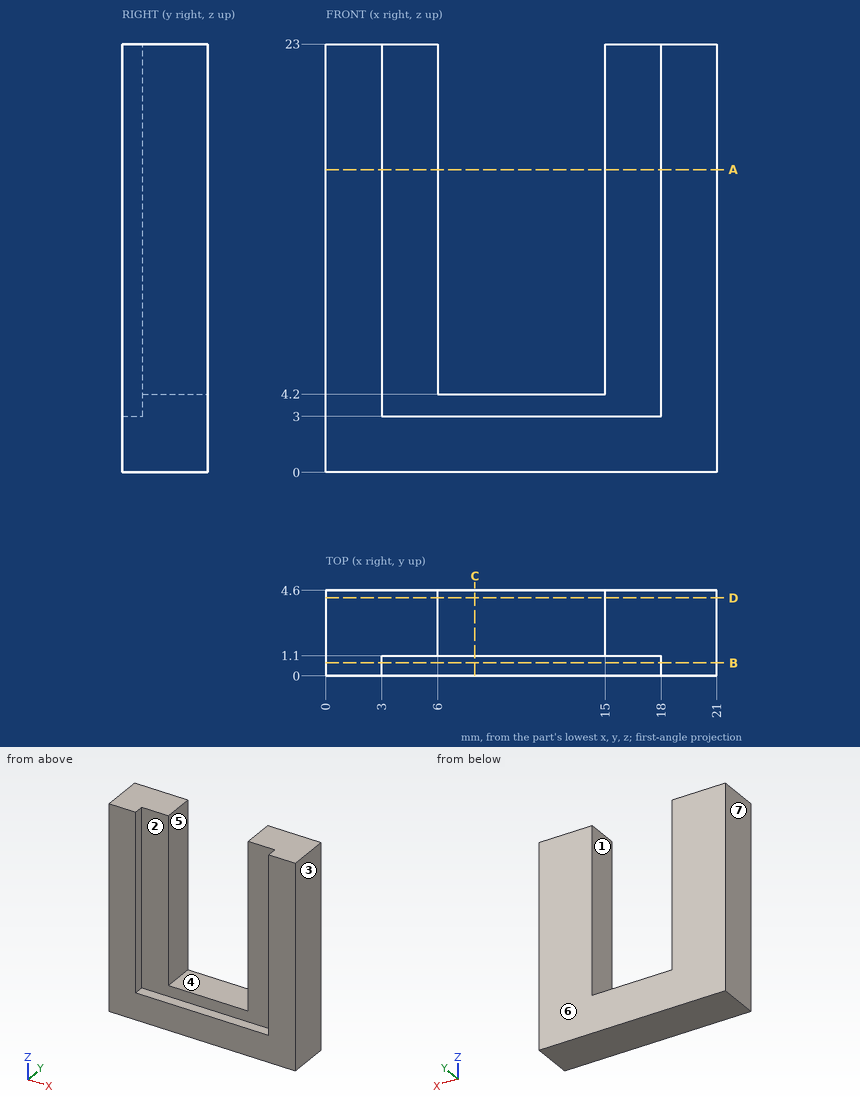
The drawing under review shows one solid part. Ordinate dimensions are in mm from its lowest x, y, z. A direction names the side the tool comes from. Coordinates: 2 decimals unless noted, no trailing zeros. Write each loop counter-clockwise with the first axis right and the second up, starting at its lowest first coordinate (ties: lowest second). Pieces come first, ordered by that corner, then holes. Notation, with made-up numbers: (1.5, -39) -> (22.5, -39) arc R21 ccw to (22.5, -30) -> close; hole circle Ø3 at (-30.75, 55.25). An arc over 180 degrees is marked (long way). One line per item, written item: value. Start each with the question number.
Q1. The part is to be moulded in two halves that separate along X. For the marked faces 4, 5, 6 and 7, say which applies: +X half, -X half, draft (parallel to the pull), parting line (faces both ways), or undercut.
Q2. To check wall thickness, follow probe 1 along X at (y, z) = (1.25, 16.25); probe 2 along X at (y, z) = (0.35, 10.5); probe 3 along Z at (x, y) = (15.5, 0.7). State the ranges of each line that lie inside material, in increasing order.
Q3. Add section B-B, the plane y = 0.7. Give the boundary of the cut face in (x, z), then the cut area to 3 significant figures.
Q4. Add section C-C, the plane x = 8. Give the boundary of the cut face in (y, z), then the cut area to 3 significant figures.
Q5. Add section D-D, the plane y = 4.2. Give the boundary of the cut face in (x, z), then the cut area to 3 significant figures.
Q6. For the marked faces 1, 2 and 3, list the 3-axis set-ups (+Z, -Z, +X, -X, +Y, -Y) from which the entire face can be reached by the end or side of a thin tool; tool diameter is ignored.
Q7. Add section A-A, the plane z = 16.25. Give the boundary of the cut face in (x, y), then the cut area to 3 significant figures.
Q8. Clearance check with flat-ended pins moving along their axes: P1, Ø1.5, axis at x = 11, y = 1.5, coming from the +Z side; P2, Ø8, axis at x = 2.5, z = 19.5, coming from the -Y side; P3, Ø0.9, axis at x = 8.5, y = 0.5, coming from the +Z side. State where each tip first meets the part, or that it passes through.
Response:
1. face 4: undercut
1. face 5: undercut
1. face 6: draft
1. face 7: -X half
2. probe 1: 0 to 6, 15 to 21
2. probe 2: 0 to 3, 18 to 21
2. probe 3: 0 to 3
3. outline: (0, 0) -> (21, 0) -> (21, 23) -> (18, 23) -> (18, 3) -> (3, 3) -> (3, 23) -> (0, 23) -> close
3. area: 183 mm²
4. outline: (0, 0) -> (4.6, 0) -> (4.6, 4.2) -> (1.1, 4.2) -> (1.1, 3) -> (0, 3) -> close
4. area: 18.0 mm²
5. outline: (0, 0) -> (21, 0) -> (21, 23) -> (15, 23) -> (15, 4.2) -> (6, 4.2) -> (6, 23) -> (0, 23) -> close
5. area: 314 mm²
6. face 1: +Z, +Y, -Y
6. face 2: +Z, -Y
6. face 3: +Z, -Z, +X, +Y, -Y
7. outline: (0, 0) -> (3, 0) -> (3, 1.1) -> (6, 1.1) -> (6, 4.6) -> (0, 4.6) -> close; (15, 1.1) -> (18, 1.1) -> (18, 0) -> (21, 0) -> (21, 4.6) -> (15, 4.6) -> close
7. area: 48.6 mm²
8. P1: z = 4.2
8. P2: y = 0
8. P3: z = 3
